Could you check a few things on this model? Use its own coordinates, in mm. Face numbers are marked on the shaded views. A direction names the side the tool comes from. Round coordinates to 2 decimals unless told otherwise and drop trailing zeros. Loops run counter-clockwise (first coordinate to the right, second up) from the corner with the lowest first, then second, coordinate; pieces in that order, holes last. Notation, with made-up numbers: (78.25, 31.5) -> (116.25, 31.5) arc R24 cw to (116.25, 46.5) -> close; hole circle Ø8 at (45, -38.5). An arc over 180 degrees is marked (long way). One line per item, written item: value.
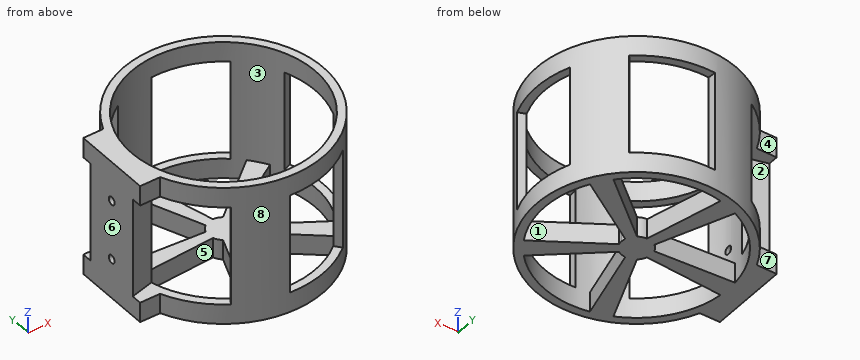
```python
from build123d import *

# Parameters (mm, degrees)
F0_R     = 46
F1_DEPTH = 70
F3_DEPTH = 10
F6_DEPTH = 50
F7_R     = 2
F8_DEPTH = 56.001


with BuildPart() as f1:
    # F0 (on Top) → F1 (new body)
    with BuildSketch(Plane.XY):
        with BuildLine():
            Line((-56, -19.5959179423), (-46, -19.5959179423))
            ThreePointArc((-46, -19.5959179423), (50, 0), (-46, 19.5959179423))
            Line((-46, 19.5959179423), (-56, 19.5959179423))
            Line((-56, 19.5959179423), (-56, -19.5959179423))
        make_face()
        Circle(F0_R, mode=Mode.SUBTRACT)
    extrude(amount=F1_DEPTH)

    # F2 (on face) → F3 (join)
    with BuildSketch(Plane(origin=(0, 0, 0), x_dir=(1, 0, 0), z_dir=(0, 0, -1))):
        with BuildLine():
            ThreePointArc((7.1900771589, -2.1337268918), (7.4221148836, -1.0780587433), (7.5, 0))
            ThreePointArc((7.5, 0), (7.4221148836, 1.0780587433), (7.1900771589, 2.1337268918))
            ThreePointArc((7.1900771589, 2.1337268918), (6.0676274578, 4.4083893922), (4.2511508974, 6.1788118637))
            ThreePointArc((4.2511508974, 6.1788118637), (2.3176274578, 7.1329238722), (0.1925611685, 7.4975276056))
            ThreePointArc((0.1925611685, 7.4975276056), (-2.3176274578, 7.1329238722), (-4.562721413, 5.9524426337))
            ThreePointArc((-4.562721413, 5.9524426337), (-6.0676274578, 4.4083893922), (-7.0710678119, 2.5))
            ThreePointArc((-7.0710678119, 2.5), (-7.5, 0), (-7.0710678119, -2.5))
            ThreePointArc((-7.0710678119, -2.5), (-6.0676274578, -4.4083893922), (-4.562721413, -5.9524426337))
            ThreePointArc((-4.562721413, -5.9524426337), (-2.3176274578, -7.1329238722), (0.1925611685, -7.4975276056))
            ThreePointArc((0.1925611685, -7.4975276056), (2.3176274578, -7.1329238722), (4.2511508975, -6.1788118637))
            ThreePointArc((4.2511508975, -6.1788118637), (6.0676274578, -4.4083893922), (7.1900771589, -2.1337268918))
        make_face()
        with BuildLine():
            ThreePointArc((-7.0710678119, -2.5), (-7.5, 0), (-7.0710678119, 2.5))
            Line((-7.0710678119, 2.5), (-45.7274534607, 5))
            ThreePointArc((-45.7274534607, 5), (-46, 0), (-45.7274534607, -5))
            Line((-45.7274534607, -5), (-7.0710678119, -2.5))
        make_face()
        with BuildLine():
            ThreePointArc((-4.562721413, 5.9524426337), (-2.3176274578, 7.1329238722), (0.1925611685, 7.4975276056))
            Line((0.1925611685, 7.4975276056), (-9.3752776474, 45.0344775593))
            ThreePointArc((-9.3752776474, 45.0344775593), (-14.2147817412, 43.7485997496), (-18.8858428103, 41.9443076155))
            Line((-18.8858428103, 41.9443076155), (-4.562721413, 5.9524426337))
        make_face()
        with BuildLine():
            ThreePointArc((4.2511508974, 6.1788118637), (6.0676274578, 4.4083893922), (7.1900771589, 2.1337268918))
            Line((7.1900771589, 2.1337268918), (39.9332132207, 22.8328377972))
            ThreePointArc((39.9332132207, 22.8328377972), (37.2147817412, 27.0381216055), (34.0553606977, 30.923007741))
            Line((34.0553606977, 30.923007741), (4.2511508974, 6.1788118637))
        make_face()
        with BuildLine():
            Line((39.9332132207, -22.8328377972), (7.1900771589, -2.1337268918))
            ThreePointArc((7.1900771589, -2.1337268918), (6.0676274578, -4.4083893922), (4.2511508975, -6.1788118637))
            Line((4.2511508975, -6.1788118637), (34.0553606977, -30.923007741))
            ThreePointArc((34.0553606977, -30.923007741), (37.2147817413, -27.0381216054), (39.9332132207, -22.8328377972))
        make_face()
        with BuildLine():
            Line((-9.3752776474, -45.0344775593), (0.1925611685, -7.4975276056))
            ThreePointArc((0.1925611685, -7.4975276056), (-2.3176274578, -7.1329238722), (-4.562721413, -5.9524426337))
            Line((-4.562721413, -5.9524426337), (-18.8858428103, -41.9443076155))
            ThreePointArc((-18.8858428103, -41.9443076155), (-14.2147817412, -43.7485997496), (-9.3752776474, -45.0344775593))
        make_face()
    extrude(amount=-F3_DEPTH)

    # F5 (on offset) → F6 (cut)
    with BuildSketch(Plane.XY.offset(10)):
        with BuildLine():
            Line((42.8084260527, 16.8356365753), (42.8084260527, -16.8356365753))
            ThreePointArc((42.8084260527, -16.8356365753), (46, 0), (42.8084260527, 16.8356365753))
        make_face()
        with BuildLine():
            ThreePointArc((42.8084260527, 16.8356365753), (46, 0), (42.8084260527, -16.8356365753))
            Line((42.8084260527, -16.8356365753), (71.2177157402, -28.0084013939))
            ThreePointArc((71.2177157402, -28.0084013939), (76.5273388005, 0), (71.2177157402, 28.0084013939))
            Line((71.2177157402, 28.0084013939), (42.8084260527, 16.8356365753))
        make_face()
        with BuildLine():
            Line((-2.7831107182, 45.9157303626), (29.2401730236, 35.5107347368))
            Line((29.2401730236, 35.5107347368), (48.645057121, 59.0770006144))
            ThreePointArc((48.645057121, 59.0770006144), (23.6482482237, 72.781824241), (-4.6300881924, 76.3871446464))
            Line((-4.6300881924, 76.3871446464), (-2.7831107182, 45.9157303626))
        make_face()
        with BuildLine():
            Line((-44.5284830709, 11.5418454071), (-24.7370052871, 38.7824776081))
            Line((-24.7370052871, 38.7824776081), (-41.1534170548, 64.519995727))
            ThreePointArc((-41.1534170548, 64.519995727), (-61.9119176239, 44.9816411442), (-74.079267614, 19.2014503011))
            Line((-74.079267614, 19.2014503011), (-44.5284830709, 11.5418454071))
        make_face()
        with BuildLine():
            Line((-24.7370052871, -38.7824776081), (-44.5284830709, -11.5418454071))
            Line((-44.5284830709, -11.5418454071), (-74.079267614, -19.2014503011))
            ThreePointArc((-74.079267614, -19.2014503011), (-61.9119176239, -44.9816411442), (-41.1534170548, -64.519995727))
            Line((-41.1534170548, -64.519995727), (-24.7370052871, -38.7824776081))
        make_face()
        with BuildLine():
            Line((29.2401730236, -35.5107347368), (-2.7831107182, -45.9157303626))
            Line((-2.7831107182, -45.9157303626), (-4.6300881924, -76.3871446464))
            ThreePointArc((-4.6300881924, -76.3871446464), (23.6482482237, -72.781824241), (48.645057121, -59.0770006144))
            Line((48.645057121, -59.0770006144), (29.2401730236, -35.5107347368))
        make_face()
    extrude(amount=F6_DEPTH, mode=Mode.SUBTRACT)

    # F7 (on Right) → F8 (cut, through all)
    with BuildSketch(Plane.YZ):
        with Locations((0, 50)):
            Circle(F7_R)
        with Locations((0, 20)):
            Circle(F7_R)
    extrude(amount=-F8_DEPTH, mode=Mode.SUBTRACT)


solid = f1.part
```
Item 1: If we mould it in two halves opening along X, with no side actions, what happens to the marked faces 5, 6, 7 and 8? For each: released by +X, released by -X, zero draft, split by the parting line, or undercut.
Output:
face 5: undercut
face 6: released by -X
face 7: zero draft
face 8: split by the parting line
Item 2: If we section it at B-B on z = 38.5: List the corners of the cut face in (x, y) for me, plus the area to 3 significant figures.
Output:
outline: (-56, -14.52) -> (-44.53, -11.54) arc R46 cw to (-44.53, 11.54) -> (-56, 14.52) -> close; (-26.89, -42.15) arc R50 ccw to (-3.03, -49.91) -> (-2.78, -45.92) arc R46 cw to (-24.74, -38.78) -> close; (-26.89, 42.15) -> (-24.74, 38.78) arc R46 cw to (-2.78, 45.92) -> (-3.03, 49.91) arc R50 ccw to start; (29.24, -35.51) -> (31.78, -38.6) arc R50 ccw to (46.53, -18.3) -> (42.81, -16.84) arc R46 cw to start; (29.24, 35.51) arc R46 cw to (42.81, 16.84) -> (46.53, 18.3) arc R50 ccw to (31.78, 38.6) -> close
area: 666 mm²
Item 3: For the marked faces 1, 2, 3 and 4, which set-ups out of +Z, -Z, +X, -X, +Y, -Y let a thin tool reach every point of the face, with its end or its side?
Output:
face 1: +Z, -Z
face 2: +X, +Y
face 3: +Z
face 4: +Z, -Z, -X, +Y
Item 4: I need wall thicknesses on line 1 (Z direction, x = -52, y = 0); line 2 (Z direction, x = -32.5, y = 37.5); line 3 (Z direction, x = -47, y = 1). Which ranges of each line are inside material? Lowest first, please. Write a range as from..to.
Output:
line 1: z = 0..18, 22..48, 52..70
line 2: z = 0..10, 60..70
line 3: z = 0..18.27, 21.73..48.27, 51.73..70
Item 5: Will these pins go through, and if not, where does the flat tip stop? pin 1 Ø5 at (x, z) = (-17, 30.5) entering from -Y; pin 2 Ø5 at (x, z) = (-51, 3) entering from +Y; pin 3 Ø15.5 at (x, y) = (-40.5, 33) entering from -Z; pin 4 Ø2 at (y, z) = (37, 47.5) entering from +X.
Output:
pin 1: stops at y = -47.85
pin 2: stops at y = 19.6
pin 3: stops at z = 0
pin 4: stops at x = 34.7
Item 6: If we section it at A-A on z = 20: List the corners of the cut face in (x, y) for me, plus the area to 3 significant figures.
Output:
outline: (-56, -14.52) -> (-44.53, -11.54) arc R46 cw to (-45.96, -2) -> (-56, -2) -> close; (-56, 2) -> (-45.96, 2) arc R46 cw to (-44.53, 11.54) -> (-56, 14.52) -> close; (-26.89, -42.15) arc R50 ccw to (-3.03, -49.91) -> (-2.78, -45.92) arc R46 cw to (-24.74, -38.78) -> close; (-26.89, 42.15) -> (-24.74, 38.78) arc R46 cw to (-2.78, 45.92) -> (-3.03, 49.91) arc R50 ccw to start; (29.24, -35.51) -> (31.78, -38.6) arc R50 ccw to (46.53, -18.3) -> (42.81, -16.84) arc R46 cw to start; (29.24, 35.51) arc R46 cw to (42.81, 16.84) -> (46.53, 18.3) arc R50 ccw to (31.78, 38.6) -> close
area: 626 mm²
Item 7: If we section it at C-C on x = -23: List the corners of the cut face in (y, z) for me, plus the area to 3 significant figures.
Output:
outline: (-44.4, 0) -> (-39.84, 0) -> (-39.84, 70) -> (-44.4, 70) -> close; (-3.53, 0) -> (3.53, 0) -> (3.53, 10) -> (-3.53, 10) -> close; (39.84, 0) -> (44.4, 0) -> (44.4, 70) -> (39.84, 70) -> close
area: 709 mm²
Item 8: If we section it at D-D on y = -33: List the corners of the cut face in (x, z) for me.
Output:
outline: (-37.56, 0) -> (-32.05, 0) -> (-32.05, 10) -> (-37.56, 10) -> close; (-37.56, 60) -> (-32.05, 60) -> (-32.05, 70) -> (-37.56, 70) -> close; (-15.33, 0) -> (-6.31, 0) -> (-6.31, 10) -> (-15.33, 10) -> close; (32.05, 0) -> (37.56, 0) -> (37.56, 70) -> (32.05, 70) -> close
